Could you check a few things on this model? Use its own coordinates, in mm. A direction names the side the tool comes from. Give positions to 0.01 mm unless a question says otherwise; leave off trailing zeros. Loops run counter-clockwise (first coordinate to the right, second up) from the corner with the lowest first, then second, coordinate; pieces in that order, holes last. Notation, with made-up numbers: (4.5, 49.5) - (47.5, 49.5) arc R28 cw to (47.5, 82.5) - close; hole circle Ø11 at (56, 0.25). An arc over 180 degrees is marked (long way). Use CSV: the item, a comma, the result in double quotes.
from build123d import *

# Parameters (mm, degrees)
SKETCH1_R               = 43.5
BOSS_EXTRUDE1_DEPTH     = 30
SKETCH2_R               = 42
CUT_EXTRUDE1_DEPTH      = 1
CUT_EXTRUDE1_DEPTH_BACK = 25
SKETCH6_W               = 1.5
SKETCH6_H               = 54
BOSS_EXTRUDE4_DEPTH     = 80
SKETCH7_W               = 54
SKETCH7_H               = 6.26870776
CUT_EXTRUDE2_DEPTH      = 15.49497474
SKETCH8_W               = 54
SKETCH8_H               = 3.87063504
CUT_EXTRUDE3_DEPTH      = 15.49497474
CUT_EXTRUDE5_REACH      = 16.495
SKETCH9_R               = 1.6
SKETCH10_W              = 2
SKETCH10_H              = 28.990761916
BOSS_EXTRUDE5_DEPTH     = 67
CUT_EXTRUDE6_REACH      = 16.562
SKETCH11_W              = 28.990761916
SKETCH11_H              = 6.298062211
CUT_EXTRUDE7_REACH      = 16.562
SKETCH12_W              = 2.183875445
SKETCH12_H              = 60.701937789
CUT_EXTRUDE8_REACH      = 16.562
SKETCH13_R              = 1.35


with BuildPart() as part:
    # Sketch1 → Boss-Extrude1 (new body)
    with BuildSketch(Plane(origin=(0, 0, 0), x_dir=(1, 0, 0), z_dir=(0, 1, 0))):
        Circle(SKETCH1_R)
    extrude(amount=BOSS_EXTRUDE1_DEPTH)

    # Sketch2 → Cut-Extrude1 (cut, two sides)
    with BuildSketch(Plane(origin=(0, 30, 0), x_dir=(1, 0, 0), z_dir=(0, 1, 0))) as cut_extrude1_sk:
        Circle(SKETCH2_R)
    extrude(amount=CUT_EXTRUDE1_DEPTH, mode=Mode.SUBTRACT)
    extrude(cut_extrude1_sk.sketch, amount=-CUT_EXTRUDE1_DEPTH_BACK, mode=Mode.SUBTRACT)

    # Sketch6 → Boss-Extrude4 (add)
    with BuildSketch(Plane(origin=(0, 5, 0), x_dir=(1, 0, 0), z_dir=(0, 1, 0))):
        with Locations((-29.75502526, -0.820126033)):
            Rectangle(SKETCH6_W, SKETCH6_H)
    extrude(amount=BOSS_EXTRUDE4_DEPTH)

    # Sketch7 → Cut-Extrude2 (cut, through all)
    with BuildSketch(Plane(origin=(-29.00502526, 0, 0), x_dir=(0, 0, -1), z_dir=(1, 0, 0))):
        with Locations((-0.820126033, 81.86564612)):
            Rectangle(SKETCH7_W, SKETCH7_H)
    extrude(amount=-CUT_EXTRUDE2_DEPTH, mode=Mode.SUBTRACT)

    # Sketch8 → Cut-Extrude3 (cut, through all)
    with BuildSketch(Plane(origin=(-29.00502526, 0, 0), x_dir=(0, 0, -1), z_dir=(1, 0, 0))):
        with Locations((-0.820126033, 76.79597472)):
            Rectangle(SKETCH8_W, SKETCH8_H)
    extrude(amount=-CUT_EXTRUDE3_DEPTH, mode=Mode.SUBTRACT)

    # Sketch9 → Cut-Extrude5 (cut, up to next)
    with BuildSketch(Plane(origin=(-29.00502526, 0, 0), x_dir=(0, 0, -1), z_dir=(1, 0, 0)), mode=Mode.PRIVATE) as cut_extrude5_sk1:
        with Locations((-25.320126033, 60.8606572)):
            Circle(SKETCH9_R)
    cut_extrude5_tool1 = extrude(cut_extrude5_sk1.sketch, amount=-CUT_EXTRUDE5_REACH, mode=Mode.PRIVATE) & part.part
    add(cut_extrude5_tool1.solids().sort_by_distance((-29.005025, 60.860657, 25.320126))[0], mode=Mode.SUBTRACT)
    # Sketch9 → Cut-Extrude5 (cut, up to next)
    with BuildSketch(Plane(origin=(-29.00502526, 0, 0), x_dir=(0, 0, -1), z_dir=(1, 0, 0)), mode=Mode.PRIVATE) as cut_extrude5_sk2:
        with Locations((22.979873967, 59.2606572)):
            Circle(SKETCH9_R)
    cut_extrude5_tool2 = extrude(cut_extrude5_sk2.sketch, amount=-CUT_EXTRUDE5_REACH, mode=Mode.PRIVATE) & part.part
    add(cut_extrude5_tool2.solids().sort_by_distance((-29.005025, 59.260657, -22.979874))[0], mode=Mode.SUBTRACT)
    # Sketch9 → Cut-Extrude5 (cut, up to next)
    with BuildSketch(Plane(origin=(-29.00502526, 0, 0), x_dir=(0, 0, -1), z_dir=(1, 0, 0)), mode=Mode.PRIVATE) as cut_extrude5_sk3:
        with Locations((7.679873967, 8.4606572)):
            Circle(SKETCH9_R)
    cut_extrude5_tool3 = extrude(cut_extrude5_sk3.sketch, amount=-CUT_EXTRUDE5_REACH, mode=Mode.PRIVATE) & part.part
    add(cut_extrude5_tool3.solids().sort_by_distance((-29.005025, 8.460657, -7.679874))[0], mode=Mode.SUBTRACT)
    # Sketch9 → Cut-Extrude5 (cut, up to next)
    with BuildSketch(Plane(origin=(-29.00502526, 0, 0), x_dir=(0, 0, -1), z_dir=(1, 0, 0)), mode=Mode.PRIVATE) as cut_extrude5_sk4:
        with Locations((-20.220126033, 8.4606572)):
            Circle(SKETCH9_R)
    cut_extrude5_tool4 = extrude(cut_extrude5_sk4.sketch, amount=-CUT_EXTRUDE5_REACH, mode=Mode.PRIVATE) & part.part
    add(cut_extrude5_tool4.solids().sort_by_distance((-29.005025, 8.460657, 20.220126))[0], mode=Mode.SUBTRACT)

    # Sketch10 → Boss-Extrude5 (add)
    with BuildSketch(Plane(origin=(0, 5, 0), x_dir=(1, 0, 0), z_dir=(0, 1, 0))):
        with Locations((29.938305356, 10.104953072)):
            Rectangle(SKETCH10_W, SKETCH10_H)
    extrude(amount=BOSS_EXTRUDE5_DEPTH)

    # Sketch11 → Cut-Extrude6 (cut, up to next)
    with BuildSketch(Plane.ZY.offset(-28.938305356), mode=Mode.PRIVATE) as cut_extrude6_sk1:
        with Locations((-10.104953072, 68.850968894)):
            Rectangle(SKETCH11_W, SKETCH11_H)
    cut_extrude6_tool1 = extrude(cut_extrude6_sk1.sketch, amount=-CUT_EXTRUDE6_REACH, mode=Mode.PRIVATE) & part.part
    add(cut_extrude6_tool1.solids().sort_by_distance((28.938305, 68.850969, -10.104953))[0], mode=Mode.SUBTRACT)

    # Sketch12 → Cut-Extrude7 (cut, up to next)
    with BuildSketch(Plane.ZY.offset(-28.938305356), mode=Mode.PRIVATE) as cut_extrude7_sk1:
        with Locations((3.298490164, 35.350968894)):
            Rectangle(SKETCH12_W, SKETCH12_H)
    cut_extrude7_tool1 = extrude(cut_extrude7_sk1.sketch, amount=-CUT_EXTRUDE7_REACH, mode=Mode.PRIVATE) & part.part
    add(cut_extrude7_tool1.solids().sort_by_distance((28.938305, 35.350969, 3.29849))[0], mode=Mode.SUBTRACT)

    # Sketch13 → Cut-Extrude8 (cut, up to next)
    with BuildSketch(Plane.ZY.offset(-28.938305356), mode=Mode.PRIVATE) as cut_extrude8_sk1:
        with Locations((-22.15033403, 62.75)):
            Circle(SKETCH13_R)
    cut_extrude8_tool1 = extrude(cut_extrude8_sk1.sketch, amount=-CUT_EXTRUDE8_REACH, mode=Mode.PRIVATE) & part.part
    add(cut_extrude8_tool1.solids().sort_by_distance((28.938305, 62.75, -22.150334))[0], mode=Mode.SUBTRACT)
    # Sketch13 → Cut-Extrude8 (cut, up to next)
    with BuildSketch(Plane.ZY.offset(-28.938305356), mode=Mode.PRIVATE) as cut_extrude8_sk2:
        with Locations((-0.85033403, 62.75)):
            Circle(SKETCH13_R)
    cut_extrude8_tool2 = extrude(cut_extrude8_sk2.sketch, amount=-CUT_EXTRUDE8_REACH, mode=Mode.PRIVATE) & part.part
    add(cut_extrude8_tool2.solids().sort_by_distance((28.938305, 62.75, -0.850334))[0], mode=Mode.SUBTRACT)
    # Sketch13 → Cut-Extrude8 (cut, up to next)
    with BuildSketch(Plane.ZY.offset(-28.938305356), mode=Mode.PRIVATE) as cut_extrude8_sk3:
        with Locations((-22.15033403, 7.45)):
            Circle(SKETCH13_R)
    cut_extrude8_tool3 = extrude(cut_extrude8_sk3.sketch, amount=-CUT_EXTRUDE8_REACH, mode=Mode.PRIVATE) & part.part
    add(cut_extrude8_tool3.solids().sort_by_distance((28.938305, 7.45, -22.150334))[0], mode=Mode.SUBTRACT)
    # Sketch13 → Cut-Extrude8 (cut, up to next)
    with BuildSketch(Plane.ZY.offset(-28.938305356), mode=Mode.PRIVATE) as cut_extrude8_sk4:
        with Locations((-0.85033403, 7.45)):
            Circle(SKETCH13_R)
    cut_extrude8_tool4 = extrude(cut_extrude8_sk4.sketch, amount=-CUT_EXTRUDE8_REACH, mode=Mode.PRIVATE) & part.part
    add(cut_extrude8_tool4.solids().sort_by_distance((28.938305, 7.45, -0.850334))[0], mode=Mode.SUBTRACT)


solid = part.part
1) I need wall thicknesses on line 1 along X through (y, z) = (58, -5); line 2 along Z through (x, y) = (30, 7); line 3 along X through (y, z) = (20, -9.5). Which ranges of each line are inside material? Lowest first, please.
Answer below:
line 1,"x = -30.51 to -29.01, 28.94 to 30.94"
line 2,"z = -31.5 to -29.39, -24.6 to -23.42, -20.88 to -2.12, 0.42 to 2.21, 29.39 to 31.5"
line 3,"x = -42.45 to -40.91, -30.51 to -29.01, 28.94 to 30.94, 40.91 to 42.45"
2) Suppose I cut it at C-C (x = 0). Please give me the cut outline in (y, z).
Answer below:
outline,"(0, -43.5) - (30, -43.5) - (30, -42) - (5, -42) - (5, 42) - (30, 42) - (30, 43.5) - (0, 43.5) - close"
3) Suppose I cut it at D-D (z = -35). Please give me the cut outline in (x, y).
Answer below:
outline,"(-25.83, 0) - (25.83, 0) - (25.83, 30) - (23.22, 30) - (23.22, 5) - (-23.22, 5) - (-23.22, 30) - (-25.83, 30) - close"
4) We'd pull the mould along Z, two halves only. Please class faces 1 (the flat face through (-23, 30, -36)), 2 (the flat face through (-1, 5, -1)), 3 (the flat face through (-29.005, 39, 1)), 4 (the cylindrical face through (-5.66, 14.79, -43.13)): +Z half, -Z half, draft (parallel to the pull), parting line (faces both ways), or undercut.
Answer below:
face 1,"draft"
face 2,"undercut"
face 3,"undercut"
face 4,"parting line"
5) Suppose I cut it at B-B (y = 27). Please give me the cut outline in (x, z).
Answer below:
outline,"circle Ø87 at (0, 0); (-30.51, -26.18) - (-29.01, -26.18) - (-29.01, 27.82) - (-30.51, 27.82) - close; (28.94, -24.6) - (30.94, -24.6) - (30.94, 2.21) - (28.94, 2.21) - close; hole circle Ø84 at (0, 0)"
6) Suppose I cut it at A-A (y = 53). Please give me the cut outline in (x, z).
Answer below:
outline,"(-30.51, -26.18) - (-29.01, -26.18) - (-29.01, 27.82) - (-30.51, 27.82) - close; (28.94, -24.6) - (30.94, -24.6) - (30.94, 2.21) - (28.94, 2.21) - close"
7) I'm going to push flat-ended pins straight in: P1, Ø0.6, axis at x = 30, y = 30, coming from the +Z side; P2, Ø1.2, axis at x = -29.5, y = 46, coming from the -Z side; P3, Ø5, axis at y = 60.86, z = 25.32, coming from the -X side (3 decimals); P4, Ø1.5, axis at x = 2, y = 32.5, coming from the -Z side. Where does each tip first touch, or does it pass through?
Answer below:
P1,"stops at z = 31.78"
P2,"stops at z = -26.18"
P3,"stops at x = -30.505"
P4,"passes through"
8) Which directions (+Z, -Z, +X, -X, +Y, -Y) give clear straight access to the entire face, cutting with the end or side of a thin tool? Please do faces 5 (the cylindrical face through (29.9, 7.5, -2.2)), 6 (the flat face through (28.938, 35, -11)), 7 (the cylindrical face through (29.92, 61.43, -1.14)).
Answer below:
face 5,"none"
face 6,"+Y"
face 7,"+X"
